from build123d import *

# Parameters (mm, degrees)
SKETCH_1_R      = 2
SKETCH_1_R_2    = 2.08
SKETCH_1_R_3    = 5
EXTRUDE_2_DEPTH = 2


with BuildPart() as part:
    # 草图1 → 凸台-拉伸2 (new body)
    with BuildSketch(Plane.XY):
        with BuildLine():
            ThreePointArc((-24, -15), (0, -20.769061509), (24, -15))
            Line((24, -15), (30, -15))
            Line((30, -15), (30, -18))
            Line((30, -18), (37, -18))
            Line((37, -18), (37, -15))
            Line((37, -15), (41, -15))
            Line((41, -15), (41, -9))
            Line((41, -9), (38, -9))
            Line((38, -9), (38, -4))
            Line((38, -4), (41, -4))
            Line((41, -4), (41, 4))
            Line((41, 4), (38, 4))
            Line((38, 4), (38, 9))
            Line((38, 9), (41, 9))
            Line((41, 9), (41, 15))
            Line((41, 15), (37, 15))
            Line((37, 15), (37, 18))
            Line((37, 18), (30, 18))
            Line((30, 18), (30, 15))
            Line((30, 15), (24, 15))
            ThreePointArc((24, 15), (0, 20.769061509), (-24, 15))
            Line((-24, 15), (-30, 15))
            Line((-30, 15), (-30, 18))
            Line((-30, 18), (-37, 18))
            Line((-37, 18), (-37, 15))
            Line((-37, 15), (-41, 15))
            Line((-41, 15), (-41, 9))
            Line((-41, 9), (-38, 9))
            Line((-38, 9), (-38, 4))
            Line((-38, 4), (-41, 4))
            Line((-41, 4), (-41, -4))
            Line((-41, -4), (-38, -4))
            Line((-38, -4), (-38, -9))
            Line((-38, -9), (-41, -9))
            Line((-41, -9), (-41, -15))
            Line((-41, -15), (-37, -15))
            Line((-37, -15), (-37, -18))
            Line((-37, -18), (-30, -18))
            Line((-30, -18), (-30, -15))
            Line((-30, -15), (-24, -15))
        make_face()
        with Locations((7.5, 12.990381057)):
            Circle(SKETCH_1_R, mode=Mode.SUBTRACT)
        with Locations((0, 13.53)):
            Circle(SKETCH_1_R_2, mode=Mode.SUBTRACT)
        with Locations((-7.5, 12.990381057)):
            Circle(SKETCH_1_R, mode=Mode.SUBTRACT)
        with Locations((-15, 0)):
            Circle(SKETCH_1_R, mode=Mode.SUBTRACT)
        with Locations((-11.717323713, -6.765)):
            Circle(SKETCH_1_R_2, mode=Mode.SUBTRACT)
        with Locations((-7.5, -12.990381057)):
            Circle(SKETCH_1_R, mode=Mode.SUBTRACT)
        with Locations((7.5, -12.990381057)):
            Circle(SKETCH_1_R, mode=Mode.SUBTRACT)
        with Locations((11.717323713, -6.765)):
            Circle(SKETCH_1_R_2, mode=Mode.SUBTRACT)
        with Locations((15, 0)):
            Circle(SKETCH_1_R, mode=Mode.SUBTRACT)
        Circle(SKETCH_1_R_3, mode=Mode.SUBTRACT)
    extrude(amount=EXTRUDE_2_DEPTH)


solid = part.part
Source: CAD feature listing. Evaluate the final solid. Frame: model axes, mm. A direction names the side the tool comes from. Coordinates: 2 decimals unless noted, no trailing zeros. Write each loop counter-clockwise with the first axis right and the second up, starting at its lowest first coordinate (ties: lowest second). Pieces come first, ordered by that corner, then holes. Notation, with made-up numbers: M -2.75,-11 L 51.25,-11 A21 ccw 51.25,19 Z; hole C -14.75,33.5 d6. An arc over 180 degrees is marked long. Use a Markdown table: item, result.
1) Mould query, pull axis X, two halves, no side actions, for faces 1 (the cylindrical face through (10.067, -8.031, 0.986)), 2 (the flat face through (37, 16, 1)), 3 (the flat face through (-41, -12, 1)), 4 (the flat face through (-39, 4, 1)). Classes: pulls with the +X half, pulls with the -X half, needs draft (parallel to the pull), parting line crosses it, or undercut.
Conclusion:
| item | result |
|---|---|
| face 1 | undercut |
| face 2 | pulls with the +X half |
| face 3 | pulls with the -X half |
| face 4 | needs draft |
2) Section B-B, the plane y = 0. Output: boundary loops of the cut face in (x, z), then the cut area to 3 significant figures.
Conclusion:
| item | result |
|---|---|
| outline | M -41,0 L -17,0 L -17,2 L -41,2 Z; M -13,0 L -5,0 L -5,2 L -13,2 Z; M 5,0 L 13,0 L 13,2 L 5,2 Z; M 17,0 L 41,0 L 41,2 L 17,2 Z |
| area | 128 mm^2 |
3) Reachability of faces 5 (the flat face through (-39, 15, 1)), 6 (the flat face through (-37, -16, 1)), 7 (the flat face through (34, 18, 1)) from +Z, -Z, +X, -X, +Y, -Y: full face, straight path, thin tool, end or side. Return the list, or none.
Conclusion:
| item | result |
|---|---|
| face 5 | +Z, -Z, -X, +Y |
| face 6 | +Z, -Z, -X, -Y |
| face 7 | +Z, -Z, +X, +Y |
4) First-contact query: pin 1 Ø0.6 at (y, z) = (-6.5, 1) entering from -X; pin 2 Ø0.6 at (x, z) = (-39.5, 1) entering from +Y; pin 3 Ø0.6 at (y, z) = (-16.5, 1) entering from +X. Flat tips, straight axial feed; report the tip coordinate or a pass-through.
Conclusion:
| item | result |
|---|---|
| pin 1 | stops at x = -38 |
| pin 2 | stops at y = 15 |
| pin 3 | stops at x = 37 |
5) Section D-D, the plane y = 17. Output: boundary loops of the cut face in (x, z), then the cut area to 3 significant figures.
Conclusion:
| item | result |
|---|---|
| outline | M -37,0 L -30,0 L -30,2 L -37,2 Z; M -19.59,0 L 19.59,0 L 19.59,2 L -19.59,2 Z; M 30,0 L 37,0 L 37,2 L 30,2 Z |
| area | 106 mm^2 |
6) Section A-A, the plane x = 0. Output: boundary loops of the cut face in (y, z), then the cut area to 3 significant figures.
Conclusion:
| item | result |
|---|---|
| outline | M -20.77,0 L -5,0 L -5,2 L -20.77,2 Z; M 5,0 L 11.45,0 L 11.45,2 L 5,2 Z; M 15.61,0 L 20.77,0 L 20.77,2 L 15.61,2 Z |
| area | 54.8 mm^2 |
7) Section C-C, the plane x = 15. Output: boundary loops of the cut face in (y, z).
Conclusion:
| item | result |
|---|---|
| outline | M -18.59,0 L -2,0 L -2,2 L -18.59,2 Z; M 2,0 L 18.59,0 L 18.59,2 L 2,2 Z |
8) Ray query, L1, parallel to X at y = -14, z = 0.2; L2, parallel to X at y = 14, z = 1.4; L3, parallel to Y at x = -7.5, z = 1.5. Return the intervals inside material, ascending.
Conclusion:
| item | result |
|---|---|
| L1 | x = -41 to -9.23, -5.77 to 5.77, 9.23 to 41 |
| L2 | x = -41 to -9.23, -5.77 to -2.03, 2.03 to 5.77, 9.23 to 41 |
| L3 | y = -20.23 to -14.99, -10.99 to 10.99, 14.99 to 20.23 |
